from build123d import *

# Parameters (mm, degrees)
BASE_FLANGE1_DEPTH = 100
EDGE_FLANGE1_DEPTH = 197.2
EDGE_FLANGE2_DEPTH = 197.2
HOLE1_START        = -1.4
HOLE1_OUTLINE_R    = 4.5
HOLE1_OUTLINE_R_2  = 1.5
HOLE1_DEPTH        = 102.8
CUT_EXTRUDE2_REACH = 231.743
SKETCH20_R         = 1.21
CUT_EXTRUDE3_REACH = 231.743
SKETCH22_R         = 1.5
SKETCH22_R_2       = 1.87
CUT_EXTRUDE4_REACH = 231.743
SKETCH25_R         = 1.5


# Read off the part's stored shape, not the designer's step: Hole1
# Sheet-metal steps are written as plain solids
with BuildPart() as part:
    # Sketch1 → Base-Flange1 (new body)
    with BuildSketch(Plane(origin=(0, 0, 0), x_dir=(1, 0, 0), z_dir=(0, 1, 0))):
        with BuildLine():
            Line((0, 50), (0, 1.4))
            ThreePointArc((0, 1.4), (0.410050506, 0.410050506), (1.4, 0))
            Line((1.4, 0), (198.6, 0))
            ThreePointArc((198.6, 0), (199.589949494, 0.410050506), (200, 1.4))
            Line((200, 1.4), (200, 48.6))
            ThreePointArc((200, 48.6), (199.589949494, 49.589949494), (198.6, 50))
            Line((198.6, 50), (145, 50))
            Line((145, 50), (145, 49.3))
            Line((145, 49.3), (198.6, 49.3))
            ThreePointArc((198.6, 49.3), (199.094974747, 49.094974747), (199.3, 48.6))
            Line((199.3, 48.6), (199.3, 1.4))
            ThreePointArc((199.3, 1.4), (199.094974747, 0.905025253), (198.6, 0.7))
            Line((198.6, 0.7), (1.4, 0.7))
            ThreePointArc((1.4, 0.7), (0.905025253, 0.905025253), (0.7, 1.4))
            Line((0.7, 1.4), (0.7, 50))
            Line((0.7, 50), (0, 50))
        make_face()
    extrude(amount=BASE_FLANGE1_DEPTH)

    # Edge-Flange1 section (across the edge) → Edge-Flange1 (add)
    with BuildSketch(Plane(origin=(198.6, -0.7, -0.7), x_dir=(0, 1, 0), z_dir=(-1, 0, 0))):
        with BuildLine():
            Line((-0.7, 0.7), (-0.7, 49.3))
            Line((-0.7, 49.3), (0, 49.3))
            Line((0, 49.3), (0, 0.7))
            ThreePointArc((0, 0.7), (0.205025253, 0.205025253), (0.7, 0))
            Line((0.7, 0), (0.7, -0.7))
            ThreePointArc((0.7, -0.7), (-0.289949494, -0.289949494), (-0.7, 0.7))
        make_face()
    extrude(amount=EDGE_FLANGE1_DEPTH)

    # Edge-Flange2 section (across the edge) → Edge-Flange2 (add)
    with BuildSketch(Plane(origin=(1.4, 100.7, -0.7), x_dir=(0, -1, 0), z_dir=(1, 0, 0))):
        with BuildLine():
            Line((-0.7, 0.7), (-0.7, 49.3))
            Line((-0.7, 49.3), (0, 49.3))
            Line((0, 49.3), (0, 0.7))
            ThreePointArc((0, 0.7), (0.205025253, 0.205025253), (0.7, 0))
            Line((0.7, 0), (0.7, -0.7))
            ThreePointArc((0.7, -0.7), (-0.289949494, -0.289949494), (-0.7, 0.7))
        make_face()
    extrude(amount=EDGE_FLANGE2_DEPTH)

    # Hole1 outline → Hole1 (cut)
    with BuildSketch(Plane(origin=(0, 0, 0), x_dir=(1, 0, 0), z_dir=(0, 1, 0)).offset(HOLE1_START)):
        with Locations((51.4, 36)):
            Circle(HOLE1_OUTLINE_R)
        with Locations((51.4, 26)):
            Circle(HOLE1_OUTLINE_R_2)
        with Locations((51.4, 46)):
            Circle(HOLE1_OUTLINE_R_2)
    extrude(amount=HOLE1_DEPTH, mode=Mode.SUBTRACT)

    # Sketch20 → Cut-Extrude2 (cut, up to next)
    with BuildSketch(Plane(origin=(0, 0, -50), x_dir=(-1, 0, 0), z_dir=(0, 0, -1)), mode=Mode.PRIVATE) as cut_extrude2_sk1:
        with Locations((-160, 57.75)):
            Circle(SKETCH20_R)
    cut_extrude2_tool1 = extrude(cut_extrude2_sk1.sketch, amount=-CUT_EXTRUDE2_REACH, mode=Mode.PRIVATE) & part.part
    # Sketch20 → Cut-Extrude2 (cut, up to next)
    with BuildSketch(Plane(origin=(0, 0, -50), x_dir=(-1, 0, 0), z_dir=(0, 0, -1)), mode=Mode.PRIVATE) as cut_extrude2_sk2:
        with Locations((-160, 42.25)):
            Circle(SKETCH20_R)
    cut_extrude2_tool2 = extrude(cut_extrude2_sk2.sketch, amount=-CUT_EXTRUDE2_REACH, mode=Mode.PRIVATE) & part.part
    add(cut_extrude2_tool1.solids().sort_by_distance((160, 57.75, -50))[0], mode=Mode.SUBTRACT)
    add(cut_extrude2_tool2.solids().sort_by_distance((160, 42.25, -50))[0], mode=Mode.SUBTRACT)

    # Sketch22 → Cut-Extrude3 (cut, up to next)
    with BuildSketch(Plane.XY, mode=Mode.PRIVATE) as cut_extrude3_sk1:
        with Locations((16.4, 50)):
            Circle(SKETCH22_R)
    cut_extrude3_tool1 = extrude(cut_extrude3_sk1.sketch, amount=-CUT_EXTRUDE3_REACH, mode=Mode.PRIVATE) & part.part
    # Sketch22 → Cut-Extrude3 (cut, up to next)
    with BuildSketch(Plane.XY, mode=Mode.PRIVATE) as cut_extrude3_sk2:
        with Locations((46.4, 50)):
            Circle(SKETCH22_R)
    cut_extrude3_tool2 = extrude(cut_extrude3_sk2.sketch, amount=-CUT_EXTRUDE3_REACH, mode=Mode.PRIVATE) & part.part
    # Sketch22 → Cut-Extrude3 (cut, up to next)
    with BuildSketch(Plane.XY, mode=Mode.PRIVATE) as cut_extrude3_sk3:
        with Locations((66.6, 50)):
            Circle(SKETCH22_R_2)
    cut_extrude3_tool3 = extrude(cut_extrude3_sk3.sketch, amount=-CUT_EXTRUDE3_REACH, mode=Mode.PRIVATE) & part.part
    # Sketch22 → Cut-Extrude3 (cut, up to next)
    with BuildSketch(Plane.XY, mode=Mode.PRIVATE) as cut_extrude3_sk4:
        with Locations((183.6, 50)):
            Circle(SKETCH22_R_2)
    cut_extrude3_tool4 = extrude(cut_extrude3_sk4.sketch, amount=-CUT_EXTRUDE3_REACH, mode=Mode.PRIVATE) & part.part
    add(cut_extrude3_tool1.solids().sort_by_distance((16.4, 50, 0))[0], mode=Mode.SUBTRACT)
    add(cut_extrude3_tool2.solids().sort_by_distance((46.4, 50, 0))[0], mode=Mode.SUBTRACT)
    add(cut_extrude3_tool3.solids().sort_by_distance((66.6, 50, 0))[0], mode=Mode.SUBTRACT)
    add(cut_extrude3_tool4.solids().sort_by_distance((183.6, 50, 0))[0], mode=Mode.SUBTRACT)

    # Sketch25 → Cut-Extrude4 (cut, up to next)
    with BuildSketch(Plane.XY, mode=Mode.PRIVATE) as cut_extrude4_sk1:
        with Locations((190.38, 2.56)):
            Circle(SKETCH25_R)
    cut_extrude4_tool1 = extrude(cut_extrude4_sk1.sketch, amount=-CUT_EXTRUDE4_REACH, mode=Mode.PRIVATE) & part.part
    # Sketch25 → Cut-Extrude4 (cut, up to next)
    with BuildSketch(Plane.XY, mode=Mode.PRIVATE) as cut_extrude4_sk2:
        with Locations((162.44, 2.56)):
            Circle(SKETCH25_R)
    cut_extrude4_tool2 = extrude(cut_extrude4_sk2.sketch, amount=-CUT_EXTRUDE4_REACH, mode=Mode.PRIVATE) & part.part
    # Sketch25 → Cut-Extrude4 (cut, up to next)
    with BuildSketch(Plane.XY, mode=Mode.PRIVATE) as cut_extrude4_sk3:
        with Locations((195.46, 54.63)):
            Circle(SKETCH25_R)
    cut_extrude4_tool3 = extrude(cut_extrude4_sk3.sketch, amount=-CUT_EXTRUDE4_REACH, mode=Mode.PRIVATE) & part.part
    # Sketch25 → Cut-Extrude4 (cut, up to next)
    with BuildSketch(Plane.XY, mode=Mode.PRIVATE) as cut_extrude4_sk4:
        with Locations((147.2, 53.36)):
            Circle(SKETCH25_R)
    cut_extrude4_tool4 = extrude(cut_extrude4_sk4.sketch, amount=-CUT_EXTRUDE4_REACH, mode=Mode.PRIVATE) & part.part
    add(cut_extrude4_tool1.solids().sort_by_distance((190.38, 2.56, 0))[0], mode=Mode.SUBTRACT)
    add(cut_extrude4_tool2.solids().sort_by_distance((162.44, 2.56, 0))[0], mode=Mode.SUBTRACT)
    add(cut_extrude4_tool3.solids().sort_by_distance((195.46, 54.63, 0))[0], mode=Mode.SUBTRACT)
    add(cut_extrude4_tool4.solids().sort_by_distance((147.2, 53.36, 0))[0], mode=Mode.SUBTRACT)


solid = part.part
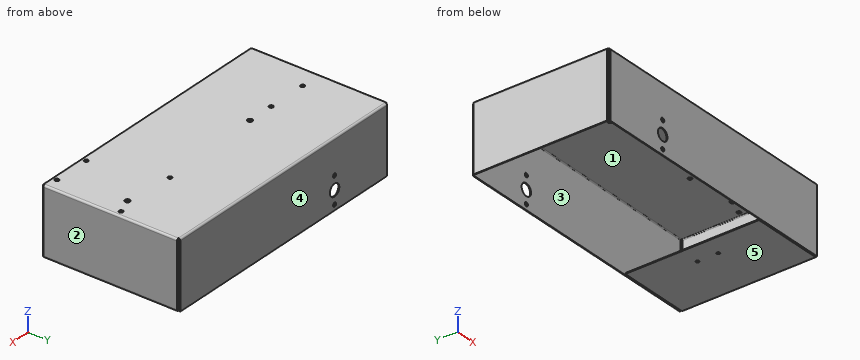
Geometry: final body of the model. Coordinates: model frame, mm. Face numbers are marked on the shaded views. A direction names the side the tool comes from. Coordinates: 2 decimals unless noted, no trailing zeros. Order: outer loops, then holes, each group sorted by start corner. A loop starts at its lowest first (then second) coordinate and runs counter-clockwise, first axis right, second up.
1) Section C-C (y = 74.5). Return loops of the section in (x, z).
Result sheet:
outline: (0, -50) - (0.7, -50) - (0.7, -1.4) arc R0.7 cw to (1.4, -0.7) - (198.6, -0.7) arc R0.7 cw to (199.3, -1.4) - (199.3, -48.6) arc R0.7 cw to (198.6, -49.3) - (145, -49.3) - (145, -50) - (198.6, -50) arc R1.4 ccw to (200, -48.6) - (200, -1.4) arc R1.4 ccw to (198.6, 0) - (1.4, 0) arc R1.4 ccw to (0, -1.4) - close
2) Ray query, probe 1 along Y at (x, z) = (160, -49.75); probe 2 along Y at (x, z) = (40.5, -19.5); probe 3 along X at (y, z) = (101.25, -46). Return the intervals inside material, ascending.
Result sheet:
probe 1: y = -1.4 to -0.7, 0 to 41.04, 43.46 to 56.54, 58.96 to 100, 100.7 to 101.4
probe 2: y = -1.4 to -0.7, 100.7 to 101.4
probe 3: x = 1.4 to 49.9, 52.9 to 198.6
3) Set-up query: the marked faces 1 and 2. Return all of +Z, -Z, +X, -X, +Y, -Y with unobstructed straight access to the full face (end or side cutting, diameter ignored); none if empty.
Result sheet:
face 1: none
face 2: +Z, -Z, +X, +Y, -Y
4) Section B-B (x = 167.5). Return loops of the section in (y, z), then the cut area to 3 significant figures.
Result sheet:
outline: (-1.4, -50) - (-0.7, -50) - (-0.7, -1.4) arc R0.7 cw to (0, -0.7) - (100, -0.7) arc R0.7 cw to (100.7, -1.4) - (100.7, -50) - (101.4, -50) - (101.4, -1.4) arc R1.4 ccw to (100, 0) - (0, 0) arc R1.4 ccw to (-1.4, -1.4) - close; (0, -50) - (100, -50) - (100, -49.3) - (0, -49.3) - close
area: 210 mm2
5) Draft query along Y for the marked faces 3, 4 and 5. Return one class per face: released by +Y, released by -Y, zero draft, split by the parting line, or undercut.
Result sheet:
face 3: undercut
face 4: released by +Y
face 5: zero draft
6) First-contact query: P1, Ø8, axis at x = 51.4, z = -36, coming from the -Y side (1 decimal); P2, Ø5, axis at x = 51.4, z = -26, coming from the -Y side; P3, Ø0.7, axis at x = 0.5, z = -21.5, coming from the -Y side. Flat tips, straight axial feed; report the tip coordinate or a pass-through.
Result sheet:
P1: passes through
P2: stops at y = -1.4
P3: stops at y = 0
7) Section A-A (z = -12.5). Return loops of the section in (x, y).
Result sheet:
outline: (0, 0) - (0.7, 0) - (0.7, 100) - (0, 100) - close; (1.4, -1.4) - (198.6, -1.4) - (198.6, -0.7) - (1.4, -0.7) - close; (1.4, 100.7) - (198.6, 100.7) - (198.6, 101.4) - (1.4, 101.4) - close; (199.3, 0) - (200, 0) - (200, 100) - (199.3, 100) - close
8) Section D-D (x = 62). Return loops of the section in (y, z), then the cut area to 3 significant figures.
Result sheet:
outline: (-1.4, -50) - (-0.7, -50) - (-0.7, -1.4) arc R0.7 cw to (0, -0.7) - (100, -0.7) arc R0.7 cw to (100.7, -1.4) - (100.7, -50) - (101.4, -50) - (101.4, -1.4) arc R1.4 ccw to (100, 0) - (0, 0) arc R1.4 ccw to (-1.4, -1.4) - close
area: 140 mm2
